Autodesk Inventor part; units mm, degrees
ref_plane "YZ Plane" through (0, 0, 0) normal (1, 0, 0) x (0, 1, 0)
ref_plane "XZ Plane" through (0, 0, 0) normal (0, 1, 0) x (-1, 0, 0)
ref_plane "XY Plane" through (0, 0, 0) normal (0, 0, 1) x (1, 0, 0)
sketch "Skizze1" plane through (0, 0, 0) normal (0, 1, 0) x (-1, 0, 0)
  line L0 (19.5, -25.5) -> (-19.5, -25.5)
  line L1 (-19.5, -25.5) -> (-19.5, 25.5)
  line L2 (-19.5, 25.5) -> (19.5, 25.5)
  line L3 (19.5, 25.5) -> (19.5, -25.5)
  line L4 (0, -35.7) -> (0, 35.7)
  line L5 (27.3, 0) -> (-27.3, 0)
  circle A0 centre (17, -23) radius 1.5
  circle A1 centre (-17, -23) radius 1.5
  circle A2 centre (17, 23) radius 1.5
  circle A3 centre (-17, 23) radius 1.5
  line L6 (15.5, 13.5) -> (-15.5, 13.5)
  line L7 (-15.5, 13.5) -> (-15.5, 20.5)
  line L8 (-15.5, 20.5) -> (15.5, 20.5)
  line L9 (15.5, 20.5) -> (15.5, 13.5)
  line L10 (16.5, 12.5) -> (1.5, 12.5)
  line L11 (1.5, 12.5) -> (1.5, -7.5)
  line L12 (1.5, -7.5) -> (16.5, -7.5)
  line L13 (16.5, -7.5) -> (16.5, 12.5)
  line L14 (-16.5, 12.5) -> (-1.5, 12.5)
  line L15 (-1.5, 12.5) -> (-1.5, -7.5)
  line L16 (-1.5, -7.5) -> (-16.5, -7.5)
  line L17 (-16.5, -7.5) -> (-16.5, 12.5)
  point P0 (0, 0)
  dimension "d0" = 39
  dimension "d1" = 51
  dimension "d2" = 3
  dimension "d3" = 2.5
  dimension "d4" = 2.5
  dimension "d5" = 7
  dimension "d6" = 5
  dimension "d7" = 31
  dimension "d8" = 15
  dimension "d9" = 20
  dimension "d19" = 3
  dimension "d20" = 13
extrude "Extrusion1" add sketch "Skizze1" along normal blind 1
extrude "Extrusion2" add sketch "Skizze1" along normal blind 10 contours L6 L7 L8 L4 | L4 L8 L9 L6
extrude "Extrusion3" add sketch "Skizze1" along normal blind 15 contours L13 L12 L11 L5 | L5 L11 L10 L13 | L15 L16 L17 L5 | L5 L17 L14 L15
chamfer "Fase1" distance 1.5 angle 45 4 edges at (0, 10, 20.5) (15.5, 10, 17) (0, 10, 13.5) (-15.5, 10, 17)
properties part number "Relais"
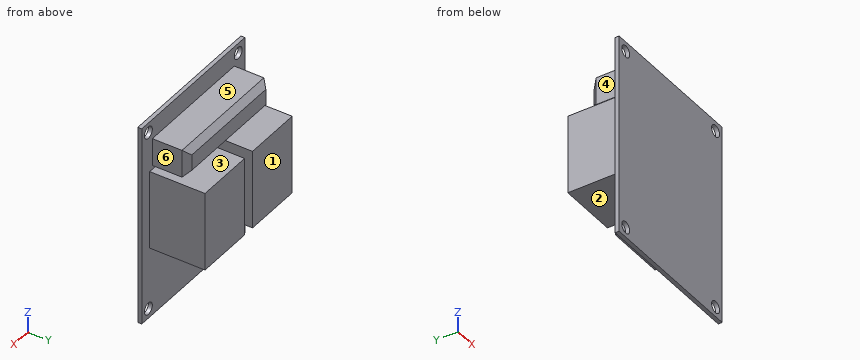
Here's how the part is built. I have some questions about the finished solid (model axes, mm). Face numbers are marked on the shaded views. A direction names the side the tool comes from. Give positions to 0.01 mm unless a question says otherwise; leave off trailing zeros. Loops run counter-clockwise (first coordinate to the right, second up) from the corner with the lowest first, then second, coordinate; pieces in that order, holes last. Notation, with made-up numbers: (4, -33) -> (59, -33) arc R17 ccw to (59, -17) -> close; hole circle Ø7 at (-16, -26.5). An arc over 180 degrees is marked (long way). Answer as a JSON object with one key per item and string values. Group by question number.
Item 1: Imagine slicing it at A-A on y = 7.25. Write out the boundary of the cut face in (x, z), then the cut area to 3 significant figures.
Item 2: Thinking about a two-plate mould opening in Z: for the marked faces 1, 2 and 3, which applies, pulls with the +Z half, pulls with the -Z half, needs draft (parallel to the pull), parting line crosses it, or undercut?
Item 3: On a 3-axis mill with a long thin cutter (end or side, diameter ignored), from which of +Z, -Z, +X, -X, +Y, -Y can I reach the whole of each face in a straight line? I mean the marked faces 4, 5 and 6. Say none if no direction works.
Item 4: Imagine slicing it at C-C on y = 11.5. Write out the boundary of the cut face in (x, z), then the cut area to 3 significant figures.
Item 5: I need wall thicknesses on L1, parallel to Z at x = -17, y = 0.45; L2, parallel to Z at x = 13, y = 3.25; L3, parallel to X at y = 11.75, z = 7. Which ranges of each line are inside material? Lowest first, please.
Item 6: Imagine slicing it at B-B on z = -23. Write out the boundary of the cut face in (x, y), then the cut area to 3 significant figures.
Item 7: Imagine slicing it at D-D on z = 6.5. Write out the boundary of the cut face in (x, y).
Item 8: Will these pins go through, and if not, where does the flat tip stop? pin 1 (7 mm diameter, centred on x = 7.5, y = 7, fed in from +Z); pin 2 (7 mm diameter, centred on y = 5, z = -1.5, fed in from -X); pin 3 (6 mm diameter, centred on x = 13, y = 5.5, fed in from -Z).
Answer list:
{
 "1": {"outline": "(-16.5, -7.5) -> (-1.5, -7.5) -> (-1.5, 12.5) -> (-16.5, 12.5) -> close; (-15.5, 13.5) -> (15.5, 13.5) -> (15.5, 20.5) -> (-15.5, 20.5) -> close; (1.5, -7.5) -> (16.5, -7.5) -> (16.5, 12.5) -> (1.5, 12.5) -> close", "area": "817 mm2"},
 "2": {"face 1": "needs draft", "face 2": "pulls with the -Z half", "face 3": "undercut"},
 "3": {"face 4": "+Z, -X, +Y", "face 5": "+Z, +X, -X, +Y", "face 6": "+Z, +X, +Y"},
 "4": {"outline": "(-16.5, -7.5) -> (-1.5, -7.5) -> (-1.5, 12.5) -> (-16.5, 12.5) -> close; (1.5, -7.5) -> (16.5, -7.5) -> (16.5, 12.5) -> (1.5, 12.5) -> close", "area": "600 mm2"},
 "5": {"L1": "z = -25.5 to -24.5, -21.5 to 21.5, 24.5 to 25.5", "L2": "z = -7.5 to 12.5, 13.5 to 20.5", "L3": "x = -16.5 to -1.5, 1.5 to 16.5"},
 "6": {"outline": "(-19.5, 0) -> (-18.5, 0) -> (-18.5, 1) -> (-19.5, 1) -> close; (-15.5, 0) -> (15.5, 0) -> (15.5, 1) -> (-15.5, 1) -> close; (18.5, 0) -> (19.5, 0) -> (19.5, 1) -> (18.5, 1) -> close", "area": "33.0 mm2"},
 "7": {"outline": "(-19.5, 0) -> (19.5, 0) -> (19.5, 1) -> (16.5, 1) -> (16.5, 15) -> (1.5, 15) -> (1.5, 1) -> (-1.5, 1) -> (-1.5, 15) -> (-16.5, 15) -> (-16.5, 1) -> (-19.5, 1) -> close"},
 "8": {"pin 1": "stops at z = 20.5", "pin 2": "stops at x = -16.5", "pin 3": "stops at z = -7.5"}
}
